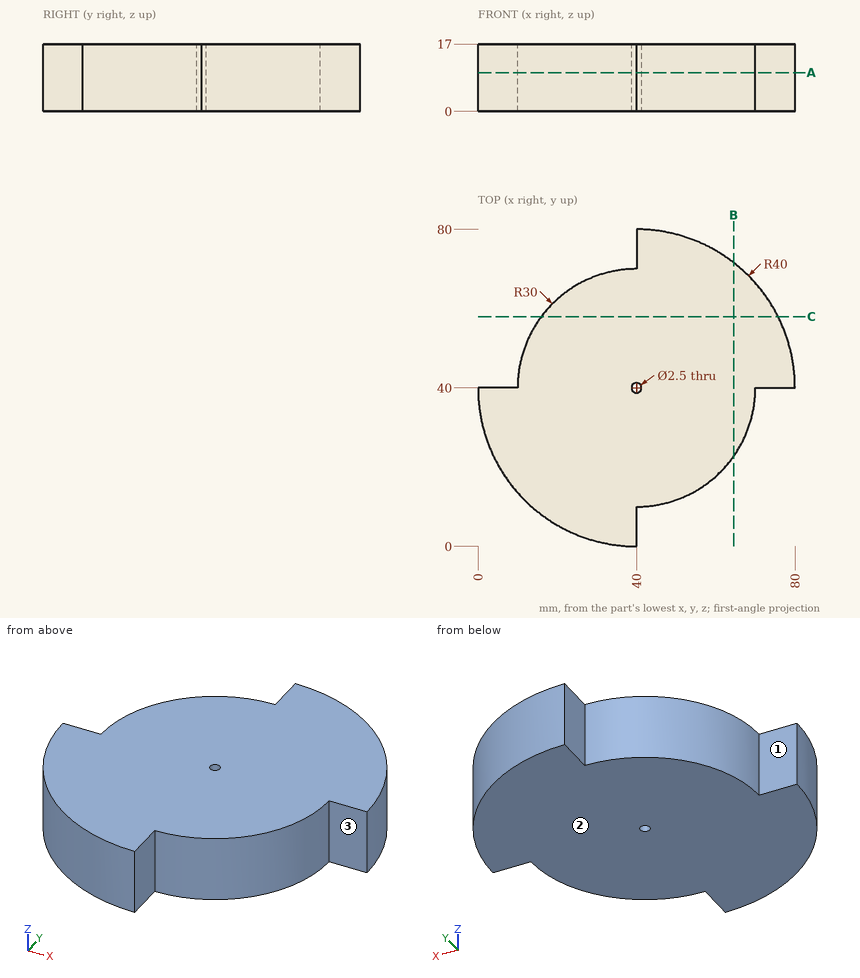
Design review of the part shown in the three views and the two pictorial views. Dimensions are in mm from the part's minimum x, y and z. A direction names the side the tool comes from. Coordinates: 2 decimals unless noted, no trailing zeros. Write each loop counter-clockwise with the first axis right and the second up, starting at its lowest first coordinate (ties: lowest second). Pieces come first, ordered by that corner, then holes.
1) We need section B-B on x = 64.5. State the section outline as (y, z) points, then the cut area to 3 significant figures.
2) Machinability: for the marked faces 1, 2 and 3, which of the approach directions +Z, -Z, +X, -X, +Y, -Y give a long, thin tool a straight path to every point of the face, cutting with its end or side? Answer none if there is none.
3) We need section C-C on y = 58. State the section outline as (x, z) points, then the cut area to 3 significant figures.
4) Clearance check with flat-ended pins moving along their axes: pin 1 Ø10 at (y, z) = (34, 11.5) entering from -X; pin 2 Ø3 at (x, y) = (40, 40) entering from -Z; pin 3 Ø8 at (y, z) = (60.5, 4.5) entering from -X; pin 4 Ø10 at (y, z) = (52, 12.5) entering from +X. State where each tip first meets the part, or that it passes through.
5) We need section A-A on z = 9.75. State the section outline as (x, y) points.
6) To check wall thickness, follow probe 1 along X at (y, z) = (5, 15.5); probe 2 along Y at (x, z) = (31.5, 1); probe 3 along X at (y, z) = (15.5, 5.5). State the ranges of each line that lie inside material, in increasing order.
Answer list:
1. outline: (22.69, 0) - (71.62, 0) - (71.62, 17) - (22.69, 17) - close
1. area: 832 mm2
2. face 1: +Z, -Z, -X, +Y
2. face 2: -Z, +X, -X, +Y, -Y
2. face 3: +Z, -Z, +X, -Y
3. outline: (16, 0) - (75.72, 0) - (75.72, 17) - (16, 17) - close
3. area: 1,020 mm2
4. pin 1: stops at x = 0.01
4. pin 2: stops at z = 0
4. pin 3: stops at x = 14.95
4. pin 4: stops at x = 79.38
5. outline: (0, 40) arc R40 ccw to (40, 0) - (40, 10) arc R30 ccw to (70, 40) - (80, 40) arc R40 ccw to (40, 80) - (40, 70) arc R30 ccw to (10, 40) - close; hole circle Ø2.5 at (40, 40)
6. probe 1: x = 20.64 to 40
6. probe 2: y = 0.91 to 68.77
6. probe 3: x = 8.38 to 57.31
